```python
from build123d import *

# Parameters (mm, degrees)
SKETCH_1_R          = 2.15
EXTRUDE_1_DEPTH     = 6
CUT_EXTRUDE_1_DEPTH = 10
FILLET_1_R          = 5
FILLET_2_R          = 3


with BuildPart() as part:
    # 草图1 → 凸台-拉伸1 (new body)
    with BuildSketch(Plane.XY):
        with BuildLine():
            Line((-52, 30), (-52, 8.75))
            Line((-52, 8.75), (-52, -8.75))
            Line((-52, -8.75), (-52, -30))
            Line((-52, -30), (-47.54, -30))
            ThreePointArc((-47.54, -30), (-44.004466094, -31.464466094), (-42.54, -35))
            Line((-42.54, -35), (-42.54, -37.5))
            ThreePointArc((-42.54, -37.5), (-38.982425028, -42.287422066), (-33.372235985, -40.262198963))
            ThreePointArc((-33.372235985, -40.262198963), (-30.171244586, -38.118753147), (-26.396349665, -38.887436588))
            ThreePointArc((-26.396349665, -38.887436588), (0, -47), (26.396349665, -38.887436588))
            ThreePointArc((26.396349665, -38.887436588), (30.171244586, -38.118753147), (33.372235985, -40.262198963))
            ThreePointArc((33.372235985, -40.262198963), (38.674773042, -42.369526686), (42.499484755, -38.135225128))
            Line((42.499484755, -38.135225128), (46.619156699, -5.971116201))
            ThreePointArc((46.619156699, -5.971116201), (47, 0), (46.619156699, 5.971116201))
            Line((46.619156699, 5.971116201), (42.499484755, 38.135225128))
            ThreePointArc((42.499484755, 38.135225128), (38.674773042, 42.369526686), (33.372235985, 40.262198963))
            ThreePointArc((33.372235985, 40.262198963), (30.171244586, 38.118753147), (26.396349665, 38.887436588))
            ThreePointArc((26.396349665, 38.887436588), (0, 47), (-26.396349665, 38.887436588))
            ThreePointArc((-26.396349665, 38.887436588), (-30.171244586, 38.118753147), (-33.372235985, 40.262198963))
            ThreePointArc((-33.372235985, 40.262198963), (-38.982425028, 42.287422066), (-42.54, 37.5))
            Line((-42.54, 37.5), (-42.54, 35))
            ThreePointArc((-42.54, 35), (-44.004466094, 31.464466094), (-47.54, 30))
            Line((-47.54, 30), (-52, 30))
        make_face()
        with Locations((-37.54, -37.5)):
            Circle(SKETCH_1_R, mode=Mode.SUBTRACT)
        with Locations((37.54, -37.5)):
            Circle(SKETCH_1_R, mode=Mode.SUBTRACT)
        with Locations((-37.54, 37.5)):
            Circle(SKETCH_1_R, mode=Mode.SUBTRACT)
        with Locations((37.54, 37.5)):
            Circle(SKETCH_1_R, mode=Mode.SUBTRACT)
    extrude(amount=EXTRUDE_1_DEPTH)

    # 草图2 → 切除-拉伸1 (cut)
    with BuildSketch(Plane.XY.offset(6)):
        with BuildLine():
            Line((-14, 44.866468548), (-14, 25.966324345))
            ThreePointArc((-14, 25.966324345), (-29.5, 0), (-14, -25.966324345))
            Line((-14, -25.966324345), (-14, -44.866468548))
            ThreePointArc((-14, -44.866468548), (6.881466199, -46.493498717), (26.396349665, -38.887436588))
            ThreePointArc((26.396349665, -38.887436588), (30.171244586, -38.118753147), (33.372235985, -40.262198963))
            ThreePointArc((33.372235985, -40.262198963), (38.674773042, -42.369526686), (42.499484755, -38.135225128))
            Line((42.499484755, -38.135225128), (46.619156699, -5.971116201))
            ThreePointArc((46.619156699, -5.971116201), (47, 0), (46.619156699, 5.971116201))
            Line((46.619156699, 5.971116201), (42.499484755, 38.135225128))
            ThreePointArc((42.499484755, 38.135225128), (38.674773042, 42.369526686), (33.372235985, 40.262198963))
            ThreePointArc((33.372235985, 40.262198963), (30.171244586, 38.118753147), (26.396349665, 38.887436588))
            ThreePointArc((26.396349665, 38.887436588), (6.881466199, 46.493498717), (-14, 44.866468548))
        make_face()
    extrude(amount=-CUT_EXTRUDE_1_DEPTH, mode=Mode.SUBTRACT)

    # 圆角1
    fillet_1_edges = [part.edges().sort_by_distance(p)[0] for p in [
        (-14, -25.966324345, 3),
        (-14, 25.966324345, 3),
    ]]
    fillet(fillet_1_edges, radius=FILLET_1_R)

    # 圆角2
    fillet_2_edges = [part.edges().sort_by_distance(p)[0] for p in [
        (-14, 44.866468548, 3),
        (-14, -44.866468548, 3),
    ]]
    fillet(fillet_2_edges, radius=FILLET_2_R)


solid = part.part
```
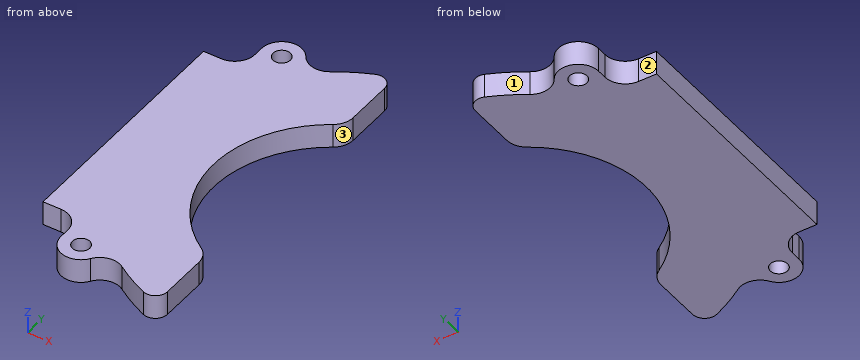
Can you work these out from the model? Positions are in its coordinate system, mm. Face numbers are marked on the shaded views. A direction names the side the tool comes from. Coordinates: 2 decimals unless noted, no trailing zeros. Loops run counter-clockwise (first coordinate to the right, second up) from the corner with the lowest first, then second, coordinate; pieces in that order, holes last.
1) Imagine slicing it at D-D on y = -12. List the corners of the cut face in (x, z) for me.
2) Imagine slicing it at B-B on z = 1.3. List the corners of the cut face in (x, y) for me.
3) For pin 1 (1.3 mm diameter, centred on x = -50, z = 4.5, fed in from +Y); pin 2 (2 mm diameter, centred on y = 36, z = 3.5, fed in from -X); pin 3 (3.5 mm diameter, centred on x = -48.5, z = 4, fed in from -Y), each with a flat end and sliding along its axis, tell me the tip position at first contact or that it passes through.
4) I need wall thicknesses on probe 1 along Y at (x, z) = (-37.54, 1.8); probe 2 along Y at (x, z) = (-39, 5.4); probe 3 along Y at (x, z) = (-19.5, 1.2). Which ranges of each line are inside material? Lowest first, please.
5) Imagine slicing it at C-C on x = -25.5. List the corners of the cut face in (y, z) for me.
6) Which directions (+Z, -Z, +X, -X, +Y, -Y) give clear straight access to the entire face, cutting with the end or side of a thin tool? Please do the marked faces 1, 2 and 3.
7) Imagine slicing it at A-A on x = -37.54. List the corners of the cut face in (y, z) for me.
Completed:
1. outline: (-52, 0) - (-26.95, 0) - (-26.95, 6) - (-52, 6) - close
2. outline: (-52, -30) - (-47.54, -30) arc R5 cw to (-42.54, -35) - (-42.54, -37.5) arc R5 ccw to (-33.37, -40.26) arc R5 cw to (-26.4, -38.89) arc R47 ccw to (-18.16, -43.35) arc R3 ccw to (-14, -40.58) - (-14, -28.8) arc R5 ccw to (-16.25, -24.62) arc R29.5 cw to (-16.25, 24.62) arc R5 ccw to (-14, 28.8) - (-14, 40.58) arc R3 ccw to (-18.16, 43.35) arc R47 ccw to (-26.4, 38.89) arc R5 cw to (-33.37, 40.26) arc R5 ccw to (-42.54, 37.5) - (-42.54, 35) arc R5 cw to (-47.54, 30) - (-52, 30) - close; hole circle Ø4.3 at (-37.54, -37.5); hole circle Ø4.3 at (-37.54, 37.5)
3. pin 1: stops at y = 30
3. pin 2: stops at x = -42.54
3. pin 3: stops at y = -30.06
4. probe 1: y = -42.5 to -39.65, -35.35 to 35.35, 39.65 to 42.5
4. probe 2: y = -42.28 to -39.08, -35.92 to 35.92, 39.08 to 42.28
4. probe 3: y = -42.76 to -22.14, 22.14 to 42.76
5. outline: (-39.48, 0) - (-14.83, 0) - (-14.83, 6) - (-39.48, 6) - close; (14.83, 0) - (39.48, 0) - (39.48, 6) - (14.83, 6) - close
6. face 1: +Z, -Z, +Y
6. face 2: +Z, -Z, -X, +Y
6. face 3: +Z, -Z, +X
7. outline: (-42.5, 0) - (-39.65, 0) - (-39.65, 6) - (-42.5, 6) - close; (-35.35, 0) - (35.35, 0) - (35.35, 6) - (-35.35, 6) - close; (39.65, 0) - (42.5, 0) - (42.5, 6) - (39.65, 6) - close
